from build123d import *

# Parameters (mm, degrees)
BOSS_EXTRUDE1_DEPTH = 21.5
SKETCH2_R           = 4.3
BOSS_EXTRUDE2_DEPTH = 8.2
SKETCH8_R           = 4.3
BOSS_EXTRUDE3_DEPTH = 3
BOSS_EXTRUDE3_TAPER = 9
SKETCH7_R           = 3.2
CUT_EXTRUDE1_DEPTH  = 31
SKETCH9_W           = 0.5
SKETCH9_H           = 1.5
BOSS_EXTRUDE4_DEPTH = 3.15


with BuildPart() as part:
    # Sketch1 → Boss-Extrude1 (new body)
    with BuildSketch(Plane.XY):
        with BuildLine():
            Line((0, 0), (15.75, 0))
            Line((15.75, 0), (15.75, 12.2))
            ThreePointArc((15.75, 12.2), (15.603553391, 12.553553391), (15.25, 12.7))
            Line((15.25, 12.7), (0.5, 12.7))
            ThreePointArc((0.5, 12.7), (0.146446609, 12.553553391), (0, 12.2))
            Line((0, 12.2), (0, 0))
        make_face()
    extrude(amount=-BOSS_EXTRUDE1_DEPTH)

    # Sketch2 → Boss-Extrude2 (add)
    with BuildSketch(Plane.XY):
        with Locations((6.43, 6.5)):
            Circle(SKETCH2_R)
    extrude(amount=BOSS_EXTRUDE2_DEPTH)

    # Sketch8 → Boss-Extrude3 (add)
    with BuildSketch(Plane(origin=(0, 0, -21.5), x_dir=(-1, 0, 0), z_dir=(0, 0, -1))):
        with Locations(Location((-6.43, 6.5, 0), (0, 0, 180))):
            Circle(SKETCH8_R)
    extrude(amount=BOSS_EXTRUDE3_DEPTH, taper=BOSS_EXTRUDE3_TAPER)

    # Sketch7 → Cut-Extrude1 (cut)
    with BuildSketch(Plane.XY.offset(8.2)):
        with Locations((6.43, 6.5)):
            Circle(SKETCH7_R)
    extrude(amount=-CUT_EXTRUDE1_DEPTH, mode=Mode.SUBTRACT)

    # Sketch9 → Boss-Extrude4 (add)
    with BuildSketch(Plane.XZ):
        with Locations((2.23, -4.75)):
            Rectangle(SKETCH9_W, SKETCH9_H)
        with Locations((13.66, -4.75)):
            Rectangle(SKETCH9_W, SKETCH9_H)
        with Locations((2.23, -17.45)):
            Rectangle(SKETCH9_W, SKETCH9_H)
        with Locations((13.66, -17.45)):
            Rectangle(SKETCH9_W, SKETCH9_H)
    extrude(amount=BOSS_EXTRUDE4_DEPTH)


solid = part.part
Read the model definition and answer for the solid it produces. Units are mm, in the model's axes. A direction names the side the tool comes from. Give positions to 0.01 mm unless a question says otherwise; leave off trailing zeros. Write each loop counter-clockwise with the first axis right and the second up, starting at its lowest first coordinate (ties: lowest second). Pieces come first, ordered by that corner, then holes. Notation, with made-up numbers: (-32, 23.25) - (6, 23.25) arc R14 ccw to (6, 43.25) - close; hole circle Ø1 at (42, 57.5). An arc over 180 degrees is marked (long way). Answer in a Markdown table with one row per item. Add a question column.
Item 1: Section B-B, the plane z = -11 is taken. Write down the section's boundary in (x, y).
Item 2: Flat-ended cylindrical pins translate along their axes: P1, Ø1.6, axis at y = -2.5, z = -4.5, coming from the +X side; P2, Ø1.2, axis at y = -2, z = -17.5, coming from the -X side; P3, Ø1.5, axis at x = 7, z = -3, coming from the -Y side. Find the tip coordinate at first contact, or state that the pin passes through.
Item 3: Section C-C, the plane x = 6.43 is taken. Write down the section's boundary in (y, z), and give its area (3 significant figures).
Item 4: Section A-A, the plane y = -0.75 is taken. Write down the section's boundary in (x, z).
Item 5: Section D-D, the plane z = 2.5 is taken. Write down the section's boundary in (x, y).
Item 6: Determine the mould class of faces 1 (the face through (6, 6, -24.5)), 2 (the face through (5.57, 10.36, -23.69)), 3 (the face through (6, 7, -22.8)) for opening direction Y: pulls with the +Y half, pulls with the -Y half, needs draft (parallel to the pull), parting line crosses it, or undercut.
Item 7: Find the intervals of material crossed by L1, parallel to Y at x = 6.43, z = -12; L2, parallel to Y at x = 6.43, z = 0.5; L3, parallel to Y at x = 14.5, z = -2, in increasing order.
Item 8: A tool of negligible diameter and unlimited length cuts with its end or side. For faces 4 (the face through (3.02, 3.88, 4.04)), 5 (the face through (2.48, -2, -5)), 6 (the face through (13.91, -2, -5)), 7 (the face through (11, 6, -21.5)), 8 (the face through (1.98, -2, -5)), from which of +Z, -Z, +X, -X, +Y, -Y can it reach the whole face along a straight path? Write none if from no direction.
Recorded:
| question | item | result |
|---|---|---|
| 1 | outline | (0, 0) - (15.75, 0) - (15.75, 12.2) arc R0.5 ccw to (15.25, 12.7) - (0.5, 12.7) arc R0.5 ccw to (0, 12.2) - close; hole circle Ø6.4 at (6.43, 6.5) |
| 2 | P1 | stops at x = 13.91 |
| 2 | P2 | stops at x = 1.98 |
| 2 | P3 | stops at y = 0 |
| 3 | outline | (0, -21.5) - (2.2, -21.5) - (2.68, -24.5) - (10.32, -24.5) - (10.8, -21.5) - (12.7, -21.5) - (12.7, 0) - (10.8, 0) - (10.8, 8.2) - (9.7, 8.2) - (9.7, -22.8) - (3.3, -22.8) - (3.3, 8.2) - (2.2, 8.2) - (2.2, 0) - (0, 0) - close |
| 3 | area | 170 mm2 |
| 4 | outline | (1.98, -18.2) - (2.48, -18.2) - (2.48, -16.7) - (1.98, -16.7) - close; (1.98, -5.5) - (2.48, -5.5) - (2.48, -4) - (1.98, -4) - close; (13.41, -18.2) - (13.91, -18.2) - (13.91, -16.7) - (13.41, -16.7) - close; (13.41, -5.5) - (13.91, -5.5) - (13.91, -4) - (13.41, -4) - close |
| 5 | outline | circle Ø8.6 at (6.43, 6.5); hole circle Ø6.4 at (6.43, 6.5) |
| 6 | face 1 | needs draft |
| 6 | face 2 | parting line crosses it |
| 6 | face 3 | undercut |
| 7 | L1 | y = 0 to 3.3, 9.7 to 12.7 |
| 7 | L2 | y = 2.2 to 3.3, 9.7 to 10.8 |
| 7 | L3 | y = 0 to 12.7 |
| 8 | face 4 | +Z |
| 8 | face 5 | +Z, -Z, -Y |
| 8 | face 6 | +Z, -Z, +X, -Y |
| 8 | face 7 | -Z |
| 8 | face 8 | +Z, -Z, -X, -Y |
